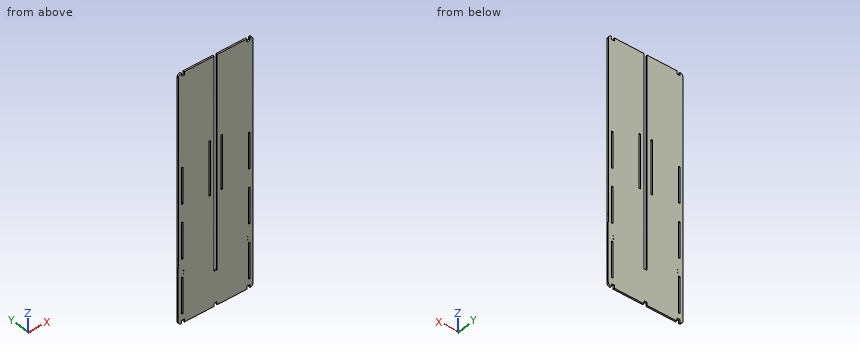
from build123d import *

# Parameters (mm, degrees)
SKETCH2_W           = 5
SKETCH2_H           = 120
BOSS_EXTRUDE1_DEPTH = 5
SKETCH3_R           = 1
SKETCH3_W           = 5
SKETCH3_H           = 180
CUT_EXTRUDE1_DEPTH  = 5
FILLET1_R           = 10
SKETCH4_W           = 10
SKETCH4_H           = 10
CUT_EXTRUDE2_DEPTH  = 10


with BuildPart() as part:
    # Sketch2 → Boss-Extrude1 (new body)
    with BuildSketch(Plane(origin=(0, 0, 0), x_dir=(1, 0, 0), z_dir=(0, 1, 0))):
        Polygon((0, 375), (0, 0), (0, -230), (10, -230), (15, -230), (117.5, -230), (117.5, 475), (127.5, 475), (127.5, -230), (230, -230), (235, -230), (245, -230), (245, -10), (245, 355), (245.3, 385), (245.3, 590), (245, 590), (0, 590), (-0.3, 590), (-0.3, 405), align=None)
        with Locations((12.5, 140)):
            Rectangle(SKETCH2_W, SKETCH2_H, mode=Mode.SUBTRACT)
        with Locations((232.5, 140)):
            Rectangle(SKETCH2_W, SKETCH2_H, mode=Mode.SUBTRACT)
        with Locations((12.5, 320)):
            Rectangle(SKETCH2_W, SKETCH2_H, mode=Mode.SUBTRACT)
        with Locations((12.5, 500)):
            Rectangle(SKETCH2_W, SKETCH2_H, mode=Mode.SUBTRACT)
        with Locations((232.5, 320)):
            Rectangle(SKETCH2_W, SKETCH2_H, mode=Mode.SUBTRACT)
        with Locations((232.5, 500)):
            Rectangle(SKETCH2_W, SKETCH2_H, mode=Mode.SUBTRACT)
    extrude(amount=BOSS_EXTRUDE1_DEPTH)

    # Sketch3 → Cut-Extrude1 (cut)
    with BuildSketch(Plane(origin=(0, 5, 0), x_dir=(1, 0, 0), z_dir=(0, 1, 0))):
        with Locations((17, 420)):
            Circle(SKETCH3_R)
        with Locations((17, 430)):
            Circle(SKETCH3_R)
        with Locations((102.5, 130)):
            Rectangle(SKETCH3_W, SKETCH3_H)
    cut_extrude1 = extrude(amount=-CUT_EXTRUDE1_DEPTH, mode=Mode.SUBTRACT)

    # Mirror1: Cut-Extrude1 across plane
    add(cut_extrude1.mirror(Plane.ZY.offset(-122.5)), mode=Mode.SUBTRACT)

    # Fillet1
    fillet1_edges = [part.edges().sort_by_distance(p)[0] for p in [
        (245, 2.5, 230),
        (0, 2.5, 230),
        (-0.3, 2.5, -590),
        (245.3, 2.5, -590),
    ]]
    fillet(fillet1_edges, radius=FILLET1_R)

    # Sketch4 → Cut-Extrude2 (cut)
    with BuildSketch(Plane(origin=(0, 5, 0), x_dir=(1, 0, 0), z_dir=(0, 1, 0))):
        with Locations((15, -225)):
            Rectangle(SKETCH4_W, SKETCH4_H)
        with Locations((230, -225)):
            Rectangle(SKETCH4_W, SKETCH4_H)
        with Locations((14.7, 585)):
            Rectangle(SKETCH4_W, SKETCH4_H)
        with Locations((230.3, 585)):
            Rectangle(SKETCH4_W, SKETCH4_H)
        with Locations((122.5, 585)):
            Rectangle(SKETCH4_W, SKETCH4_H)
    extrude(amount=-CUT_EXTRUDE2_DEPTH, mode=Mode.SUBTRACT)


solid = part.part
Input: part model. Units: mm. Frame: model coordinates. Coordinates: 2 decimals unless noted, no trailing zeros. Write each loop counter-clockwise with the first axis right and the second up, starting at its lowest first coordinate (ties: lowest second). Pieces come first, ordered by that corner, then holes. Notation, with made-up numbers: M 36.5,41.25 L 89.5,41.25 A17 ccw 89.5,60.25 Z; hole C 18.5,29.5 d6. An arc over 180 degrees is marked long. Answer as a JSON object with one key per item and string values. Group by question number.
(1) Contact query for flat-ended pins moving along their axis: P1, Ø2.5, axis at y = 2.5, z = -124.5, coming from the -X side; P2, Ø1.5, axis at x = 120.5, y = 3.5, coming from the +Z side; P3, Ø2.5, axis at y = 1.5, z = -87, coming from the +X side. Output: stop coordinate, or through.
(2) Section B-B on z = -458.5. Output: boundary loops of the cut face in (x, y).
(3) Section D-D on z = -209.5. Output: boundary loops of the cut face in (x, y), plus the area to 4 significant figures.
(4) Ray query, line 1 along X through (y, z) = (1.05, -287); line 2 along Z through (x, y) = (228, 2.35); line 3 along X through (y, z) = (3.5, -420). Return the intervals inside material, ascending. Write a range as [from, to].
(5) Section A-A on z = 101. Output: boundary loops of the cut face in (x, y), plus the area to 4 significant figures.
(6) Section C-C on y = 2.35. Give the number of separate pieces and of enclosed holes in the cut face, plus the area to 3 significant figures.
Result set:
{
 "1": {"P1": "stops at x = 0", "P2": "stops at z = -475", "P3": "stops at x = 245"},
 "2": {"outline": "M -0.3,0 L 10,0 L 10,5 L -0.3,5 Z; M 15,0 L 117.5,0 L 117.5,5 L 15,5 Z; M 127.5,0 L 230,0 L 230,5 L 127.5,5 Z; M 235,0 L 245.3,0 L 245.3,5 L 235,5 Z"},
 "3": {"outline": "M 0,0 L 100,0 L 100,5 L 0,5 Z; M 105,0 L 117.5,0 L 117.5,5 L 105,5 Z; M 127.5,0 L 140,0 L 140,5 L 127.5,5 Z; M 145,0 L 245,0 L 245,5 L 145,5 Z", "area": "1,125 mm2"},
 "4": {"line 1": "x = [0, 10], [15, 117.5], [127.5, 230], [235, 245]", "line 2": "z = [-580, -431], [-429, -421], [-419, 220]", "line 3": "x = [-0.3, 16], [18, 117.5], [127.5, 227], [229, 245.3]"},
 "5": {"outline": "M 0,0 L 117.5,0 L 117.5,5 L 0,5 Z; M 127.5,0 L 245,0 L 245,5 L 127.5,5 Z", "area": "1,175 mm2"},
 "6": {"separate pieces": "1", "enclosed holes": "12", "area": "188,000 mm2"}
}
